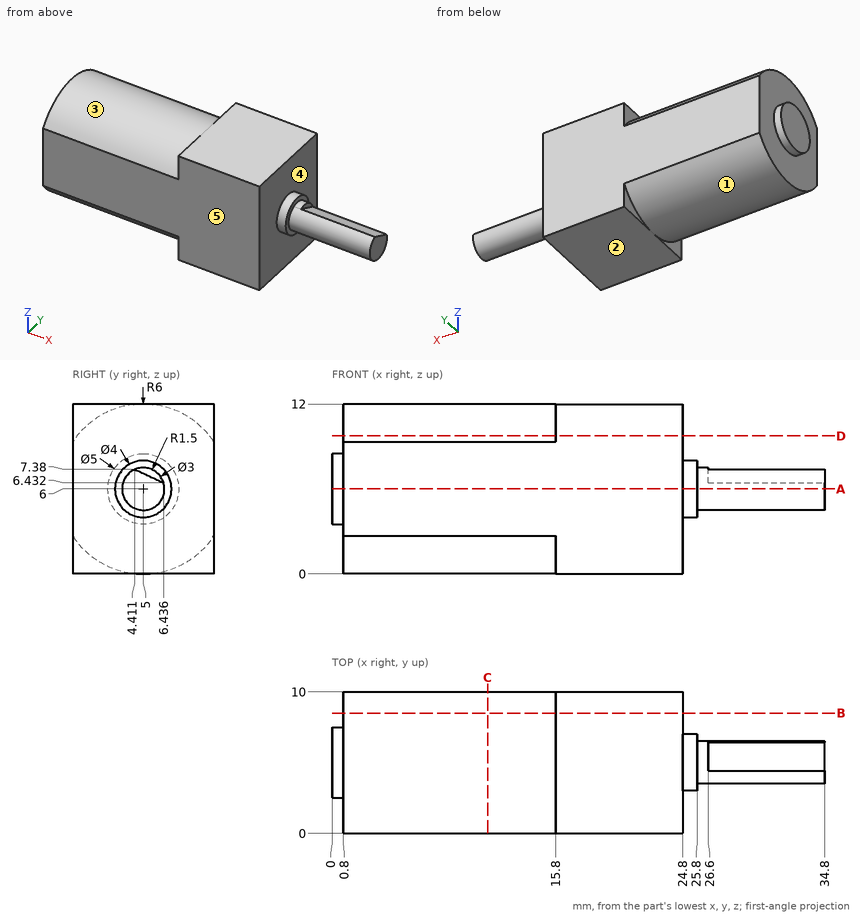
Drawing for the job (mm, zero at the part's lowest x, y, z). A direction names the side the tool comes from. Give positions to 0.01 mm unless a question says otherwise; leave off trailing zeros. Order: outer loops, then holes, each group sorted by start corner. A loop starts at its lowest first (then second) coordinate and runs counter-clockwise, first axis right, second up. Notation, with made-up numbers: M -30.75,-18 L 9.25,-18 A27 cw 9.25,20 Z; hole C 29,-21.5 d8. An arc over 180 degrees is marked long. Put each result on its own line as item: value.
Item 1: Slice it at D-D, the plane z = 9.75. Write the cut outline in (x, y).
From the geometry:
outline: M 0.8,0.32 L 15.8,0.32 L 15.8,0 L 24.8,0 L 24.8,10 L 15.8,10 L 15.8,9.68 L 0.8,9.68 Z
Item 2: Flat gauge pins, fed straight in: pin 1 Ø3 at (y, z) = (8.5, 8.5) entering from -X; pin 2 Ø3 at (y, z) = (7, 8) entering from +X; pin 3 Ø6 at (x, z) = (29.5, 7) entering from -Y. Where does each tip first touch, or does it go through?
From the geometry:
pin 1: stops at x = 0.8
pin 2: stops at x = 26.6
pin 3: stops at y = 3.5
Item 3: 3-axis set-ups, long thin cutter, end or side, ignore diameter. For the marked faces 1, 2, 3, 4 and 5: which of +Z, -Z, +X, -X, +Y, -Y reach the whole face in a straight line?
From the geometry:
face 1: -Z, -X
face 2: -Z, +X, -X, +Y, -Y
face 3: +Z, -X
face 4: +X
face 5: +Z, -Z, +X, -X, -Y
Item 4: Slice it at C-C, the plane x = 11. Write the cut outline in (y, z), plus the area to 3 significant figures.
From the geometry:
outline: M 0,2.68 A6 ccw 10,2.68 L 10,9.32 A6 ccw 0,9.32 Z
area: 104 mm2
Item 5: Probe line 1 (X direction, y = 4.5, z = 10.25); line 2 (Z direction, x = 10.5, y = 5.25) (1 decimal); line 3 (Z direction, x = 8, y = 3). List the from-to ranges inside material, lowest first. Write a range as [from, to].
From the geometry:
line 1: x = [0.8, 24.8]
line 2: z = [0, 12]
line 3: z = [0.34, 11.66]
Item 6: Slice it at A-A, the plane z = 6. Write the cut outline in (x, y), plus the area to 3 significant figures.
From the geometry:
outline: M 0,2.5 L 0.8,2.5 L 0.8,0 L 24.8,0 L 24.8,3 L 25.8,3 L 25.8,3.5 L 34.8,3.5 L 34.8,6.5 L 25.8,6.5 L 25.8,7 L 24.8,7 L 24.8,10 L 0.8,10 L 0.8,7.5 L 0,7.5 Z
area: 275 mm2
Item 7: Slice it at B-B, the plane y = 8.5. Write the cut outline in (x, z).
From the geometry:
outline: M 0.8,1.13 L 15.8,1.13 L 15.8,0 L 24.8,0 L 24.8,12 L 15.8,12 L 15.8,10.87 L 0.8,10.87 Z
